CAD build for the part. Positions are in the model's coordinates, mm. Face numbers are marked on the shaded views. A direction names the side the tool comes from. Round coordinates to 2 decimals unless told otherwise and drop trailing zeros. Order: outer loops, then holes, each group sorted by start corner. A loop starts at its lowest first (then second) coordinate and runs counter-clockwise, first axis right, second up. Notation, with made-up numbers: M -19.75,49 L 3.25,49 A22 ccw 3.25,82 Z; hole C 47,5 d9. An arc over 180 degrees is marked long. Answer as a JSON object with one key per item and string values.
```python
from build123d import *

# Parameters (mm, degrees)
SKETCH1_R           = 1.5
BOSS_EXTRUDE1_DEPTH = 5
FILLET3_R           = 1
BOSS_EXTRUDE2_START = 7.5
SKETCH4_W           = 6
SKETCH4_H           = 15
BOSS_EXTRUDE2_DEPTH = 20
SKETCH5_R           = 3
BOSS_EXTRUDE3_DEPTH = 15


with BuildPart() as part:
    # Sketch1 → Boss-Extrude1 (new body)
    with BuildSketch(Plane.XY):
        with BuildLine():
            ThreePointArc((0, 6), (-6, 0), (0, -6))
            Line((0, -6), (90, -6))
            ThreePointArc((90, -6), (96, 0), (90, 6))
            Line((90, 6), (0, 6))
        make_face()
        Circle(SKETCH1_R, mode=Mode.SUBTRACT)
        with Locations((90, 0)):
            Circle(SKETCH1_R, mode=Mode.SUBTRACT)
    extrude(amount=BOSS_EXTRUDE1_DEPTH)

    # Fillet3
    fillet3_edges = [part.edges().sort_by_distance(p)[0] for p in [
        (88.5, 0, 0),
    ]]
    fillet(fillet3_edges, radius=FILLET3_R)

    # Sketch4 → Boss-Extrude2 (add)
    with BuildSketch(Plane.XY.offset(5).offset(BOSS_EXTRUDE2_START)):
        with Locations((93, 0)):
            Rectangle(SKETCH4_W, SKETCH4_H)
    extrude(amount=-BOSS_EXTRUDE2_DEPTH)

    # Sketch5 → Boss-Extrude3 (add)
    with BuildSketch(Plane(origin=(96, 0, 0), x_dir=(0, 0, -1), z_dir=(1, 0, 0))):
        with Locations((-2.5, 0)):
            Circle(SKETCH5_R)
    extrude(amount=BOSS_EXTRUDE3_DEPTH)

    # Sketch6 → Revolve1 (revolve)
    with BuildSketch(Plane(origin=(111, 0, 0), x_dir=(0, 0, -1), z_dir=(1, 0, 0))):
        with BuildLine():
            Line((-2.5, 7.5), (-2.5, -7.5))
            ThreePointArc((-2.5, -7.5), (5, 0), (-2.5, 7.5))
        make_face()
    revolve(axis=Axis((111, 7.5, 2.5), (0, -1, 0)))


solid = part.part
```
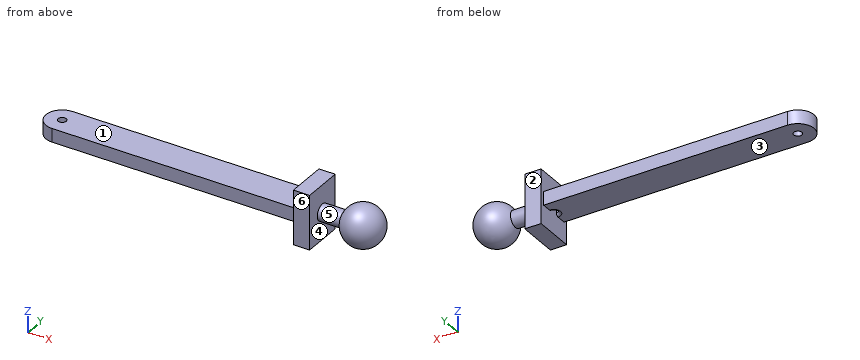
Item 1: Saw through at A-A on y = 0. List the corners of the cut face in (x, z), and give its area (3 significant figures).
Worked answers:
{"outline": "M -6,0 L -1.5,0 L -1.5,5 L -6,5 Z; M 1.5,0 L 87.5,0 A1 ccw 88.5,1 L 88.5,5 L 1.5,5 Z; M 90,-7.5 L 96,-7.5 L 96,-0.5 L 104.13,-0.5 A7.5 ccw long 104.13,5.5 L 96,5.5 L 96,12.5 L 90,12.5 Z", "area": "800 mm2"}
Item 2: Saw through at D-D on x = 101. List the corners of the cut face in (y, z).
Worked answers:
{"outline": "C 0,2.5 d6"}
Item 3: Saw through at C-C on z = 7. List the corners of the cut face in (x, y), and give its area (3 significant figures).
Worked answers:
{"outline": "M 90,-7.5 L 96,-7.5 L 96,7.5 L 90,7.5 Z; C 111,0 d12", "area": "203 mm2"}
Item 4: Saw through at B-B on z = 2.5. List the corners of the cut face in (x, y), and give its area (3 significant figures).
Worked answers:
{"outline": "M 0,-6 L 90,-6 L 90,-7.5 L 96,-7.5 L 96,-3 L 104.13,-3 A7.5 ccw long 104.13,3 L 96,3 L 96,7.5 L 90,7.5 L 90,6 L 0,6 A6 ccw Z; hole C 0,0 d3; hole M 90,-1.5 L 90,1.5 A1.5 ccw Z", "area": "1,440 mm2"}
Item 5: Wall check: line 1 along X through (y, z) = (-2.25, -6.25); line 2 along Z through (x, y) = (41, -5); line 3 along X through (y, z) = (-2.75, 4.75). Give the ranges that are in metal, low to high. Write a range as [from, to].
Worked answers:
{"line 1": "x = [90, 96]", "line 2": "z = [0, 5]", "line 3": "x = [-5.33, 96], [104.4, 117.6]"}
Item 6: Two-plate mould, pull along X, no slides. Class the marked faces 5 and 6: released by +X, released by -X, zero draft, split by the parting line, or undercut.
Worked answers:
{"face 5": "undercut", "face 6": "zero draft"}
Item 7: 3-axis set-ups, long thin cutter, end or side, ignore diameter. For the marked faces 1, 2, 3 and 4: which of +Z, -Z, +X, -X, +Y, -Y reach the whole face in a straight line?
Worked answers:
{"face 1": "+Z, -X, +Y, -Y", "face 2": "+Z, -Z, +X, -X, +Y", "face 3": "-Z, -X, +Y, -Y", "face 4": "none"}
Item 8: Drop flat-ended pins along their axis: pin 1 Ø1 at (x, z) = (41, 1.5) entering from -Y; pin 2 Ø7.5 at (y, z) = (-3, 5) entering from +X; pin 3 Ø2 at (y, z) = (-0.5, -4.5) entering from -X. Give the stop position or say it passes through.
Worked answers:
{"pin 1": "stops at y = -6", "pin 2": "stops at x = 118.5", "pin 3": "stops at x = 90"}
